```python
from build123d import *

# Parameters (mm, degrees)
BOSS_EXTRUDE1_DEPTH = 5
SKETCH2_R           = 1.5
SKETCH2_W           = 10
SKETCH2_H           = 5
SKETCH2_W_2         = 15
SKETCH2_H_2         = 40
CUT_EXTRUDE1_DEPTH  = 10
FILLET1_R           = 10
FILLET2_R           = 1
CONG_1_R            = 1


with BuildPart() as part:
    # Sketch1 → Boss-Extrude1 (new body)
    with BuildSketch(Plane.XY):
        Polygon((-50.018889855, -56.191512275), (-30.018889855, -56.191512275), (-30.018889855, -61.191512275), (-20.018889855, -61.191512275), (-20.018889855, -56.191512275), (-11.518889855, -56.191512275), (-11.518889855, -53.191512275), (-12.618889855, -53.191512275), (-12.618889855, -50.891512275), (-11.518889855, -50.891512275), (-11.518889855, -46.191512275), (-8.518889855, -46.191512275), (-8.518889855, -50.891512275), (-7.418889855, -50.891512275), (-7.418889855, -53.191512275), (-8.518889855, -53.191512275), (-8.518889855, -56.191512275), (-0.018889855, -56.191512275), (-0.018889855, -61.191512275), (9.981110145, -61.191512275), (9.981110145, -56.191512275), (29.981110145, -56.191512275), (29.981110145, -61.191512275), (40.481110145, -61.191512275), (12.481110145, -16.103821473), (12.481110145, 58.808487725), (9.981110145, 58.808487725), (9.981110145, 68.808487725), (-0.018889855, 68.808487725), (-0.018889855, 58.808487725), (-8.518889855, 58.808487725), (-8.518889855, 50.808487725), (-7.418889855, 50.808487725), (-7.418889855, 48.508487725), (-8.518889855, 48.508487725), (-8.518889855, 43.808487725), (-11.518889855, 43.808487725), (-11.518889855, 48.508487725), (-12.618889855, 48.508487725), (-12.618889855, 50.808487725), (-11.518889855, 50.808487725), (-11.518889855, 58.808487725), (-20.018889855, 58.808487725), (-20.018889855, 68.808487725), (-30.018889855, 68.808487725), (-30.018889855, 58.808487725), (-32.518889855, 58.808487725), (-32.518889855, -16.103821473), (-60.518889855, -61.191512275), (-50.018889855, -61.191512275), align=None)
    extrude(amount=BOSS_EXTRUDE1_DEPTH)

    # Sketch2 → Cut-Extrude1 (cut)
    with BuildSketch(Plane.XY.offset(5)):
        with Locations((-10.018889855, -23.691512275)):
            Circle(SKETCH2_R)
        with Locations((-25.018889855, -23.691512275)):
            Rectangle(SKETCH2_W, SKETCH2_H)
        with Locations((4.981110145, -23.691512275)):
            Rectangle(SKETCH2_W, SKETCH2_H)
        with Locations((-10.018889855, 3.808487725)):
            Rectangle(SKETCH2_W_2, SKETCH2_H_2)
    extrude(amount=-CUT_EXTRUDE1_DEPTH, mode=Mode.SUBTRACT)

    # Fillet1
    fillet1_edges = [part.edges().sort_by_distance(p)[0] for p in [
        (-32.518889855, -16.103821473, 2.5),
        (12.481110145, -16.103821473, 2.5),
    ]]
    fillet(fillet1_edges, radius=FILLET1_R)

    # Fillet2
    fillet2_edges = [part.edges().sort_by_distance(p)[0] for p in [
        (40.481110145, -61.191512275, 2.5),
        (-60.518889855, -61.191512275, 2.5),
    ]]
    fillet(fillet2_edges, radius=FILLET2_R)

    # Congé1
    cong_1_edges = [part.edges().sort_by_distance(p)[0] for p in [
        (-30.018889855, 68.808487725, 2.5),
        (-20.018889855, 68.808487725, 2.5),
        (-0.018889855, 68.808487725, 2.5),
        (9.981110145, 68.808487725, 2.5),
    ]]
    fillet(cong_1_edges, radius=CONG_1_R)


solid = part.part
```
Design review of the part built by this model. Coordinates are the model's own, in mm. A direction names the side the tool comes from. Round coordinates to 2 decimals unless told otherwise and drop trailing zeros. Order: outer loops, then holes, each group sorted by start corner. A loop starts at its lowest first (then second) coordinate and runs counter-clockwise, first axis right, second up. Notation, with made-up numbers: M 23.5,-17.75 L 70.5,-17.75 A38 cw 70.5,20.25 Z; hole C 53.5,8.25 d7. An arc over 180 degrees is marked long. Put each result on its own line as item: value.
Q1. Consider section B-B (y = 57). State the section outline as (x, z) points.
Reported:
outline: M -32.52,0 L -11.52,0 L -11.52,5 L -32.52,5 Z; M -8.52,0 L 12.48,0 L 12.48,5 L -8.52,5 Z
Q2. Consider section A-A (x = -5.5). State the section outline as (y, z) points, and give its area (3 significant figures).
Reported:
outline: M -56.19,0 L -16.19,0 L -16.19,5 L -56.19,5 Z; M 23.81,0 L 58.81,0 L 58.81,5 L 23.81,5 Z
area: 375 mm²
Q3. Insertion check: pin 1 Ø1.5 at (y, z) = (-58.5, 1.5) entering from +X; pin 2 Ø4 at (x, y) = (-10.02, -23.69) entering from +Z; pin 3 Ø2.5 at (y, z) = (45.5, 3.5) entering from -X; pin 4 Ø1.5 at (y, z) = (-24, 3.5) entering from +X. Each pin has a flat end and moves straight along its axis. Give the tip position at first contact, or say it passes through.
Reported:
pin 1: x = 39.28
pin 2: z = 5
pin 3: x = -32.52
pin 4: x = 17.85
Q4. Machinability: for faces 1 (the face through (-25, -61.192, 2)), 2 (the face through (-20.019, 63, 2)), 3 (the face through (9.981, 63, 2)), 4 (the face through (-30.019, -59, 2)), 5 (the face through (5, -26.192, 3)), which of the approach directions +Z, -Z, +X, -X, +Y, -Y give a long, thin tool a straight path to every point of the face, cutting with its end or side? Answer none if there is none.
Reported:
face 1: +Z, -Z, +X, -X, -Y
face 2: +Z, -Z, +Y
face 3: +Z, -Z, +X, +Y
face 4: +Z, -Z, -Y
face 5: +Z, -Z
Q5. Consider section C-C (y = 36.5). State the section outline as (x, z) points.
Reported:
outline: M -32.52,0 L 12.48,0 L 12.48,5 L -32.52,5 Z
Q6. Consider section D-D (x = -38). State the section outline as (y, z) points.
Reported:
outline: M -56.19,0 L -24.93,0 L -24.93,5 L -56.19,5 Z
Q7. To check wall thickness, follow line 1 (X direction, y = 8.5, z = 4.05); line 2 (Y direction, x = -28, z = 0.9); line 3 (Y direction, x = -6, z = 0.55). State the ranges of each line that lie inside material, in increasing order.
Reported:
line 1: -32.52 to -17.52, -2.52 to 12.48
line 2: -61.19 to -26.19, -21.19 to 68.81
line 3: -56.19 to -16.19, 23.81 to 58.81
Q8. Draft analysis for pull direction X (two halves, no side actions). For faces 6 (the face through (-32.913, -16.032, 2.535)), 7 (the face through (-54, -61.192, 2)), 8 (the face through (-50.019, -59, 2)), state which applies: released by +X, released by -X, zero draft, split by the parting line, or undercut.
Reported:
face 6: released by -X
face 7: zero draft
face 8: undercut
